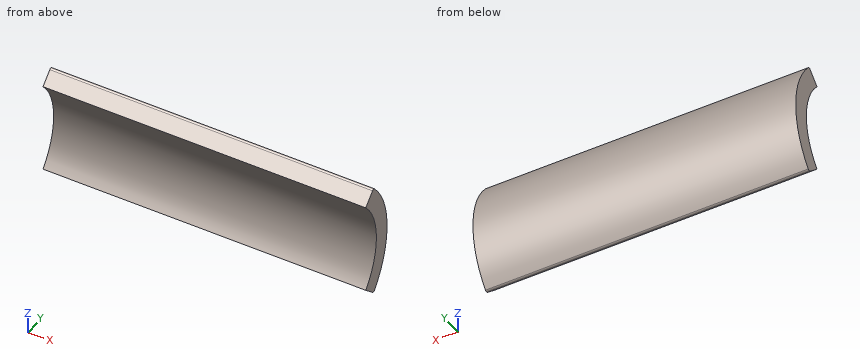
from build123d import *

# Parameters (mm, degrees)
BOSS_EXTRUDE1_DEPTH = 17.5


with BuildPart() as part:
    # Sketch1 → Boss-Extrude1 (new, symmetric)
    with BuildSketch(Plane(origin=(0, 0, 0), x_dir=(0, 0, -1), z_dir=(1, 0, 0))):
        with BuildLine():
            Line((-6.20870808, 6.716542561), (-5.036701532, 5.44867302))
            ThreePointArc((-5.036701532, 5.44867302), (0, 7.42), (5.036701532, 5.44867302))
            Line((5.036701532, 5.44867302), (6.20870808, 6.716542561))
            ThreePointArc((6.20870808, 6.716542561), (6.274777299, 6.899469771), (6.189748422, 7.074391456))
            ThreePointArc((6.189748422, 7.074391456), (0, 9.4), (-6.189748422, 7.074391456))
            ThreePointArc((-6.189748422, 7.074391456), (-6.274777299, 6.899469771), (-6.20870808, 6.716542561))
        make_face()
    extrude(amount=BOSS_EXTRUDE1_DEPTH, both=True)


solid = part.part
Geometry: final body of the model. Coordinates: model frame, mm. Give positions to 0.01 mm unless a question says otherwise; leave off trailing zeros. Loops run counter-clockwise (first coordinate to the right, second up) from the corner with the lowest first, then second, coordinate; pieces in that order, holes last. Notation, with made-up numbers: (57.25, 16.5) - (116.25, 16.5) arc R34 ccw to (116.25, 50.5) - close; hole circle Ø5 at (56, 60). An arc over 180 degrees is marked (long way). One line per question, with ' | ' between items. Start each with the question number.
(1) Section query B-B on x = -5. Return loops of the section in (y, z).
(2) Section query A-A on y = 6.25. Return loops of the section in (x, z).
(3) Ray query, line 1 (Y direction, x = 8, z = -0.25); line 2 (Z direction, x = -2, y = 6.6); line 3 (Z direction, x = -6.5, y = 5.7). Return the intervals inside material, ascending. Write a range as from..to.
(4) Section query C-C on z = -3. Return loops of the section in (x, y).
(5) Section query D-D on y = 9.1. Return loops of the section in (x, z), then the cut area to 3 significant figures.
The answers:
1) outline: (5.45, -5.04) - (6.72, -6.21) arc R0.25 ccw to (7.07, -6.19) arc R9.4 ccw to (7.07, 6.19) arc R0.25 ccw to (6.72, 6.21) - (5.45, 5.04) arc R7.42 cw to start
2) outline: (-17.5, -5.78) - (17.5, -5.78) - (17.5, -4) - (-17.5, -4) - close; (-17.5, 4) - (17.5, 4) - (17.5, 5.78) - (-17.5, 5.78) - close
3) line 1: 7.42..9.4 | line 2: -6.1..-3.39, 3.39..6.1 | line 3: -5.27..-4.75, 4.75..5.27
4) outline: (-17.5, 6.79) - (17.5, 6.79) - (17.5, 8.91) - (-17.5, 8.91) - close
5) outline: (-17.5, -2.36) - (17.5, -2.36) - (17.5, 2.36) - (-17.5, 2.36) - close | area: 165 mm2
